```python
from build123d import *

# Parameters (mm, degrees)
EXTRUDE_THIN1_DEPTH = 6.35
FILLET1_R           = 5.08
CHAMFER1_SIZE       = 2.54
SKETCH2_R           = 2.159
CUT_EXTRUDE1_DEPTH  = 47.635354958


with BuildPart() as part:
    # Sketch1 → Extrude-Thin1 (new, symmetric)
    with BuildSketch(Plane.XY):
        with BuildLine():
            Line((-45.830174209, -6.35), (-25.78993192, -6.35))
            ThreePointArc((-25.78993192, -6.35), (-24.22783192, -5.931436567), (-23.084295354, -4.7879))
            Line((-23.084295354, -4.7879), (-20.869926131, -0.9525))
            ThreePointArc((-20.869926131, -0.9525), (-20.172647737, -0.255221606), (-19.220147737, 0))
            Line((-19.220147737, 0), (19.220147737, 0))
            ThreePointArc((19.220147737, 0), (20.172647737, -0.255221606), (20.869926131, -0.9525))
            Line((20.869926131, -0.9525), (22.791001417, -4.2799))
            ThreePointArc((22.791001417, -4.2799), (23.934537984, -5.423436567), (25.496637984, -5.842))
            Line((25.496637984, -5.842), (45.536880273, -5.842))
            Line((45.536880273, -5.842), (45.536880273, -4.6228))
            Line((45.536880273, -4.6228), (25.496637984, -4.6228))
            ThreePointArc((25.496637984, -4.6228), (24.544137984, -4.367578394), (23.846859589, -3.6703))
            Line((23.846859589, -3.6703), (21.925784304, -0.3429))
            ThreePointArc((21.925784304, -0.3429), (20.782247737, 0.800636567), (19.220147737, 1.2192))
            Line((19.220147737, 1.2192), (-19.220147737, 1.2192))
            ThreePointArc((-19.220147737, 1.2192), (-20.782247737, 0.800636567), (-21.925784304, -0.3429))
            Line((-21.925784304, -0.3429), (-24.140153526, -4.1783))
            ThreePointArc((-24.140153526, -4.1783), (-24.83743192, -4.875578394), (-25.78993192, -5.1308))
            Line((-25.78993192, -5.1308), (-45.830174209, -5.1308))
            Line((-45.830174209, -5.1308), (-45.830174209, -6.35))
        make_face()
    extrude(amount=EXTRUDE_THIN1_DEPTH, both=True)

    # Fillet1
    fillet1_edges = [part.edges().sort_by_distance(p)[0] for p in [
        (45.536880273, -5.2324, -6.35),
        (45.536880273, -5.2324, 6.35),
    ]]
    fillet(fillet1_edges, radius=FILLET1_R)

    # Chamfer1
    chamfer1_edges = [part.edges().sort_by_distance(p)[0] for p in [
        (-45.830174209, -5.7404, -6.35),
        (-45.830174209, -5.7404, 6.35),
    ]]
    chamfer(chamfer1_edges, length=CHAMFER1_SIZE)

    # Sketch2 → Cut-Extrude1 (cut, through all)
    with BuildSketch(Plane(origin=(0, -4.6228, 0), x_dir=(1, 0, 0), z_dir=(0, 1, 0))):
        with Locations(Location((37.916880273, 0, 0), (0, 0, 270))):
            Circle(SKETCH2_R)
    extrude(amount=-CUT_EXTRUDE1_DEPTH, mode=Mode.SUBTRACT)


solid = part.part
```
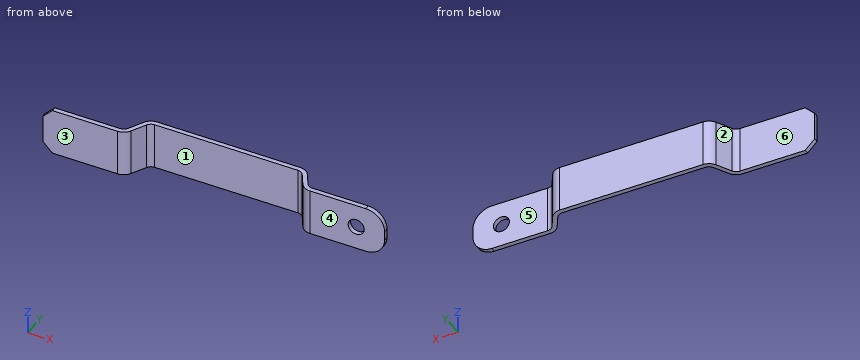
The model under review builds one solid part; all positions refer to its coordinate system, in mm. Face numbers are marked on the shaded views. A direction names the side the tool comes from. Round coordinates to 2 decimals unless told otherwise and drop trailing zeros. Write each loop counter-clockwise with the first axis right and the second up, starting at its lowest first coordinate (ties: lowest second). Pieces come first, ordered by that corner, then holes.
(1) We need section B-B on x = 37. Give the boundary of the cut face in (y, z).
(2) We need section D-D on x = 6.5. Give the boundary of the cut face in (y, z).
(3) Insertion check: pin 1 (1.5 mm diameter, centred on x = -18.5, z = 3, fed in from -Y); pin 2 (4 mm diameter, centred on x = -34.5, z = -2, fed in from +Y); pin 3 (3 mm diameter, centred on x = 31, z = -1.5, fed in from -Y). Each pin has a flat end and moves straight along its axis. Give the tip position at first contact, or say it passes through.
(4) We need section C-C on y = -2.25. Give the boundary of the cut face in (x, z), and give its area (3 significant figures).
(5) Wall thickness on L1, parallel to X at y = -4.85, z = 0; L2, parallel to Y at x = -39, z = 1; L3, parallel to X at y = -5.4, z = 0: over which ranges is each line inside the solid? List them lowest first.
(6) Mouldability with a two-part tool opening along X and no side actions: class the marked faces 1, 2 and 3 as +X half, -X half, draft (parallel to the pull), parting line (faces both ways), or undercut.
(7) Machinability: for the marked faces 4, 5 and 6, which of the approach directions +Z, -Z, +X, -X, +Y, -Y give a long, thin tool a straight path to every point of the face, cutting with its end or side? Answer none if there is none.
Findings below:
1. outline: (-5.84, -6.35) - (-4.62, -6.35) - (-4.62, -1.95) - (-5.84, -1.95) - close; (-5.84, 1.95) - (-4.62, 1.95) - (-4.62, 6.35) - (-5.84, 6.35) - close
2. outline: (0, -6.35) - (1.22, -6.35) - (1.22, 6.35) - (0, 6.35) - close
3. pin 1: stops at y = 0
3. pin 2: stops at y = -5.13
3. pin 3: stops at y = -5.84
4. outline: (-23.03, -6.35) - (-21.62, -6.35) - (-21.62, 6.35) - (-23.03, 6.35) - close; (21.62, -6.35) - (23.03, -6.35) - (23.03, 6.35) - (21.62, 6.35) - close
4. area: 35.8 mm2
5. L1: x = -24.79 to -23.12, 23.21 to 35.76, 40.08 to 45.54
5. L2: y = -6.35 to -5.13
5. L3: x = -45.83 to -23.55, 23.89 to 35.76, 40.08 to 45.54
6. face 1: undercut
6. face 2: -X half
6. face 3: draft
7. face 4: +Z, -Z, +X, -Y
7. face 5: +Z, -Z, +X, +Y
7. face 6: +Z, -Z, -X, +Y
